For this review, use the dimensioned drawing (mm, ordinates from the lowest corner) and the shaded views. A direction names the side the tool comes from. Round coordinates to 2 decimals unless told otherwise and drop trailing zeros. Write each loop counter-clockwise with the first axis right and the second up, starting at its lowest first coordinate (ties: lowest second). Pieces come first, ordered by that corner, then holes. Notation, with made-up numbers: (-16.5, -19) - (18.5, -19) arc R21 ccw to (18.5, 9) - close; hole circle Ø9 at (-29, -14). An arc over 180 degrees is marked (long way). Write each question's results on one line, items separated by ' | '.
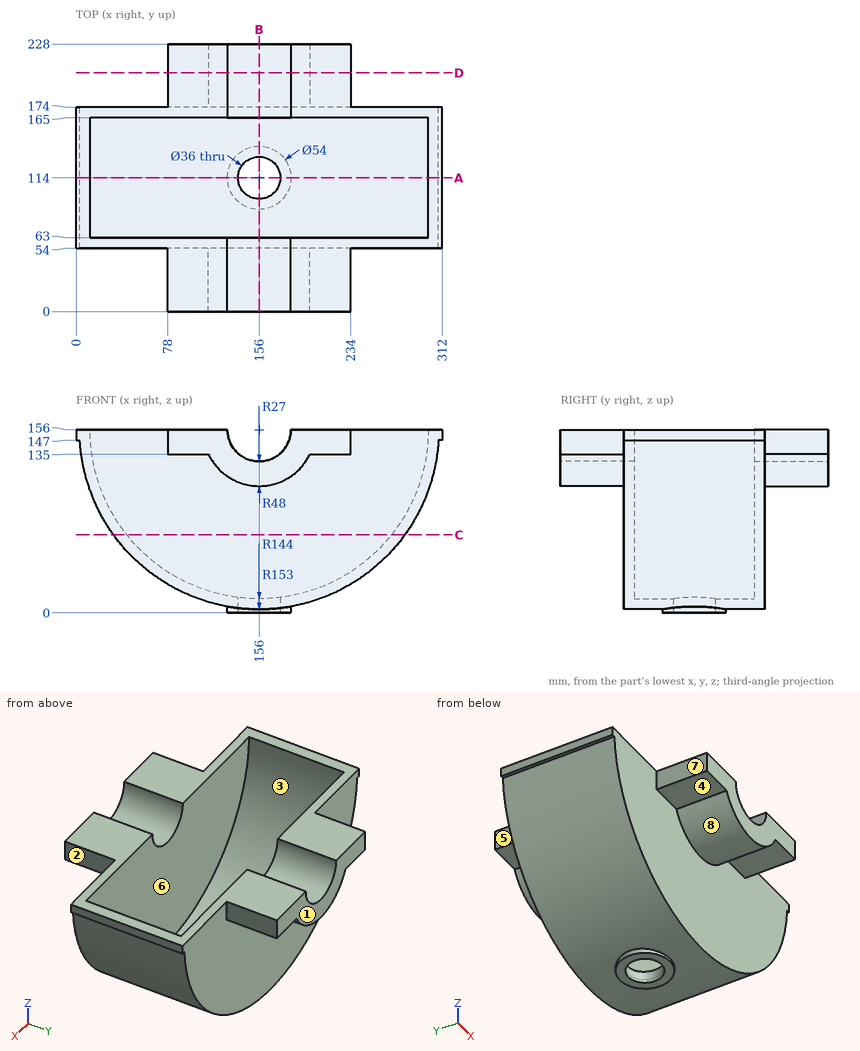
Q1. Insertion check: P1, Ø10, axis at y = 163, z = 96, coming from the +X side; P2, Ø3, axis at x = 119, y = 122, coming from the +Z side; P3, Ø10.5, axis at x = 210.5, y = 202, coming from the -Z side; P4, Ø21.5, axis at x = 156, y = 114, coming from the -Z side. Each pin has a flat end and moves straight along its axis. Give the tip position at first contact, or say it passes through.
Evaluation:
P1: stops at x = 298.77 | P2: stops at z = 17.24 | P3: stops at z = 135 | P4: passes through
Q2. For probe 1 along Y at (x, z) = (143, 79); probe 2 along Y at (x, z) = (156, 1.65); probe 3 along X at (y, z) = (114, 2.55), list the stretches that pass through material, from the lowest coordinate up.
Evaluation:
probe 1: y = 54 to 63, 165 to 174 | probe 2: y = 87 to 96, 132 to 141 | probe 3: x = 129 to 138, 174 to 183
Q3. We need section C-C (z = 66.5). State the section outline as (x, y) points.
Evaluation:
outline: (31.91, 54) - (280.09, 54) - (280.09, 174) - (31.91, 174) - close; hole (43.19, 63) - (268.81, 63) - (268.81, 165) - (43.19, 165) - close
Q4. We need section B-B (x = 156). State the section outline as (y, z) points, plus the area to 3 significant figures.
Evaluation:
outline: (0, 108) - (54, 108) - (54, 3) - (87, 3) - (87, 0) - (96, 0) - (96, 12) - (63, 12) - (63, 129) - (0, 129) - close; (132, 0) - (141, 0) - (141, 3) - (174, 3) - (174, 108) - (228, 108) - (228, 129) - (165, 129) - (165, 12) - (132, 12) - close | area: 5,180 mm^2
Q5. We need section D-D (y = 203.5). State the section outline as (x, z) points.
Evaluation:
outline: (78, 135) - (112.84, 135) arc R48 ccw to (199.16, 135) - (234, 135) - (234, 156) - (183, 156) arc R27 cw to (129, 156) - (78, 156) - close
Q6. The part is to be moulded in two halves that separate along Y. For the marked faces 1, 2 and 3, say which applies: released by +Y, released by -Y, zero draft, split by the parting line, or undercut.
Evaluation:
face 1: released by +Y | face 2: zero draft | face 3: undercut
Q7. Tool access review of the marked faces 4, 5, 6, 7 and 8: name each direction out of +Z, -Z, +X, -X, +Y, -Y from which nothing blocks a thin tool from reaching the whole face with its end or side.
Evaluation:
face 4: -Z, -X, -Y | face 5: +Z, -Z, -X, +Y | face 6: +Z | face 7: +Z, -Z, -X, -Y | face 8: -Z, -Y
Q8. We need section A-A (y = 114). State the section outline as (x, z) points.
Evaluation:
outline: (0, 147) - (3.26, 147) arc R153 ccw to (129, 5.4) - (129, 0) - (138, 0) - (138, 13.13) arc R144 cw to (12, 156) - (0, 156) - close; (174, 0) - (183, 0) - (183, 5.4) arc R153 ccw to (308.74, 147) - (312, 147) - (312, 156) - (300, 156) arc R144 cw to (174, 13.13) - close
